Read the model definition and answer for the solid it produces. Units are mm, in the model's axes. Face numbers are marked on the shaded views. A direction names the side the tool comes from. Coordinates: 2 decimals unless noted, no trailing zeros. Write each loop counter-clockwise with the first axis right and the second up, starting at its lowest first coordinate (ties: lowest second). Pieces come first, ordered by that corner, then holes. Notation, with made-up numbers: (33, -37) -> (79, -37) arc R15 ccw to (79, -33) -> close; hole circle Ø2 at (-17, 70.25). An arc over 180 degrees is marked (long way). Use CSV: the item, a comma, the result in double quotes. Start each with the question number.
from build123d import *

# Parameters (mm, degrees)
F1_DEPTH = 70
F3_DEPTH = 10


# Not quite as in the source:
# - a feature names something its author has since deleted; it is built from what else it names


with BuildPart() as f1:
    # F0 (on Right) → F1 (new body)
    with BuildSketch(Plane.YZ):
        with BuildLine():
            Line((35.0004041982, -43.4744954109), (27.8094485444, -50))
            Line((27.8094485444, -50), (-27.8090443462, -50))
            Line((-27.8090443462, -50), (-35, -43.4744954109))
            Line((-35, -43.4744954109), (-35.1477400841, 0))
            Line((-35.1477400841, 0), (-38.1477574069, 0))
            Line((-38.1477574069, 0), (-37.988001967, -47.0101745328))
            ThreePointArc((-37.988001967, -47.0101745328), (-36.2312971095, -51.2420067187), (-32, -53))
            Line((-32, -53), (32, -53))
            ThreePointArc((32, -53), (36.3403848268, -51.1600325097), (38.0115591918, -46.7519039894))
            Line((38.0115591918, -46.7519039894), (37.917284091, -19.0101948899))
            ThreePointArc((37.917284091, -19.0101948899), (38.792345044, -16.8822871618), (40.9172667684, -16))
            Line((40.9172667684, -16), (44.8968422253, -16))
            Line((44.8968422253, -16), (44.8968422253, -13))
            Line((44.8968422253, -13), (34.8968422253, -13))
            Line((34.8968422253, -13), (35.0004041982, -43.4744954109))
        make_face()
    extrude(amount=F1_DEPTH)

    # F2 (on face) → F3 (join)
    with BuildSketch(Plane.YZ.offset(70)):
        Polygon((34.9751985597, -36.0573992247), (-35.0252056385, -36.0573992247), (-35.0122565756, -39.8678341294), (-7.3888426073, -48.4471021518), (-7.3888426073, -50), (-2.3888426073, -50), (2.3879472654, -50), (7.3879472654, -50), (7.3879472654, -48.4459963804), (34.9881476226, -39.8678341294), align=None)
        Polygon((0, -46.7519039894), (-22.1652372944, -39.8678341294), (22.1494653338, -39.8678341294), align=None, mode=Mode.SUBTRACT)
    extrude(amount=-F3_DEPTH)

    # F4: F1 across plane


with BuildPart() as f1_1:
    add(f1.part)
    add(f1.part.mirror(Plane.YZ))

    # F5: F1 across plane


with BuildPart() as f1_2:
    add(f1_1.part)
    add(f1_1.part.mirror(Plane.XY))


solid = f1_2.part
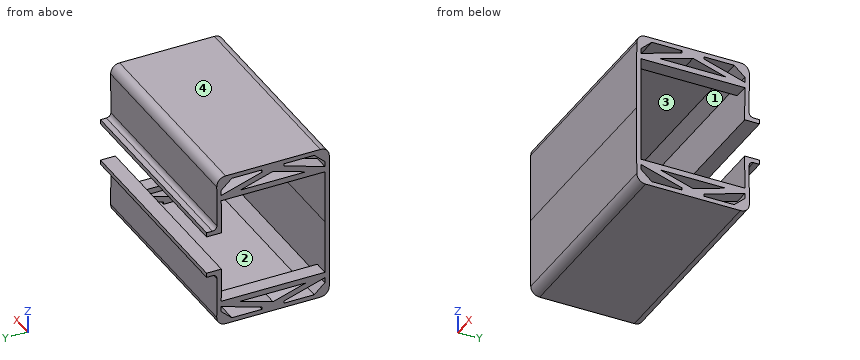
1) Section B-B, the plane x = -27.5 is taken. Give the vertices of the cut face in (y, z).
2) Find the intervals of material crossed by line 1 along X through (y, z) = (14, -37.5); line 2 along Z through (x, y) = (-13.5, -2); line 3 along Y through (x, z) = (16.5, -39), in increasing order.
3) Which of the six approach directions +Z, -Z, +X, -X, +Y, -Y give full straight-line access (tool end or side, diameter ignored) to the marked faces 3 and 4?
4) The mould has two halves that part along X. Classify the marked faces 1 and 2: pulls with the +X half, pulls with the -X half, needs draft (parallel to the pull), parting line crosses it, or undercut.
5) Section C-C, the plane z = -21.5 is taken. Give the vertices of the cut face in (x, y).
6) Section D-D, the plane y = 19.5 is taken. Count the separate pieces of the cut face and the enclosed holes in it, plus the area to 3 significant figures.
7) Section A-A, the plane z = 38 is taken. Give the vertices of the cut face in (x, y), plus the area to 3 significant figures.
8) Each of these flat-tipped pins is pushed along its axis until it touches: pin 1 (4 mm diameter, centred on x = -39, z = -42.5, fed in from +Y); pin 2 (3 mm diameter, centred on y = 23, z = -35.5, fed in from +X); pin 3 (4.5 mm diameter, centred on x = -31, y = 43.5, fed in from +Z); pin 4 (0.8 mm diameter, centred on x = -66, z = -49.5, fed in from -Y). Where does it stop, or does it pass through?
The answers:
1,outline,"(-38.15, 0) -> (-37.99, -47.01) arc R6 ccw to (-32, -53) -> (32, -53) arc R6 ccw to (38.01, -46.75) -> (37.92, -19.01) arc R3 cw to (40.92, -16) -> (44.9, -16) -> (44.9, -13) -> (34.9, -13) -> (35, -43.47) -> (27.81, -50) -> (-27.81, -50) -> (-35, -43.47) -> (-35.15, 0) -> (-35, 43.47) -> (-27.81, 50) -> (27.81, 50) -> (35, 43.47) -> (34.9, 13) -> (44.9, 13) -> (44.9, 16) -> (40.92, 16) arc R3 cw to (37.92, 19.01) -> (38.01, 46.75) arc R6 ccw to (32, 53) -> (-32, 53) arc R6 ccw to (-37.99, 47.01) -> close"
2,line 1,"x = -70 to -60, 60 to 70"
2,line 2,"z = -53 to -50, 50 to 53"
2,line 3,"y = -38.02 to -35.02, 34.99 to 37.99"
3,face 3,"none"
3,face 4,"+Z, +X, -X, +Y, -Y"
4,face 1,"needs draft"
4,face 2,"undercut"
5,outline,"(-70, -38.07) -> (70, -38.07) -> (70, -35.07) -> (-70, -35.07) -> close; (-70, 34.93) -> (70, 34.93) -> (70, 37.93) -> (-70, 37.93) -> close"
6,separate pieces,"10"
6,enclosed holes,"0"
6,area,"1,150 mm^2"
7,outline,"(-70, -38.02) -> (70, -38.02) -> (70, 37.98) -> (-70, 37.98) -> close; hole (-60, -35.02) -> (60, -35.02) -> (60, 34.98) -> (-60, 34.98) -> close"
7,area,"2,240 mm^2"
8,pin 1,"stops at y = 38"
8,pin 2,"stops at x = 70"
8,pin 3,"stops at z = 16"
8,pin 4,"stops at y = -37.61"
